from build123d import *

# Parameters (mm, degrees)
F0_W     = 195.58
F0_H     = 91.44
F1_DEPTH = 127
F2_W     = 50.8
F2_H     = 91.44
F3_DEPTH = 123.19


with BuildPart() as f1:
    # F0 (on Front) → F1 (new body)
    with BuildSketch(Plane.XZ):
        with Locations((97.79, 45.72)):
            Rectangle(F0_W, F0_H)
    extrude(amount=-F1_DEPTH)

    # F2 (on face) → F3 (cut)
    with BuildSketch(Plane.XZ):
        with Locations((25.4, 45.72)):
            Rectangle(F2_W, F2_H)
        with Locations((170.18, 45.72)):
            Rectangle(F2_W, F2_H)
    extrude(amount=-F3_DEPTH, mode=Mode.SUBTRACT)


solid = f1.part
Check sheet for the modelled part. Datum: model origin and axes. Units: mm. A direction names the side the tool comes from. Round coordinates to 2 decimals unless told otherwise and drop trailing zeros. Order: outer loops, then holes, each group sorted by start corner. A loop starts at its lowest first (then second) coordinate and runs counter-clockwise, first axis right, second up.
Q1. Depth check by flat-ended pin: P1, Ø15, axis at x = 31, z = 28, coming from the -Y side; P2, Ø4, axis at y = 40, z = 35.5, coming from the -X side. Enter the tip coordinate at first touch or a pass-through.
Filled sheet:
P1: stops at y = 123.19
P2: stops at x = 50.8
Q2. Scan lines: L1, parallel to Y at x = 152, z = 73.5; L2, parallel to X at y = 94, z = 65.5. Record each from-to range of solid material in increasing order.
Filled sheet:
L1: y = 123.19 to 127
L2: x = 50.8 to 144.78
Q3. Cross-section at C-C, the plane x = 169.5. Enter the section's corners in (y, z), plus the area to 3 significant figures.
Filled sheet:
outline: (123.19, 0) - (127, 0) - (127, 91.44) - (123.19, 91.44) - close
area: 348 mm2
Q4. Cross-section at A-A, the plane z = 29.5. Enter the section's corners in (x, y), plus the area to 3 significant figures.
Filled sheet:
outline: (0, 123.19) - (50.8, 123.19) - (50.8, 0) - (144.78, 0) - (144.78, 123.19) - (195.58, 123.19) - (195.58, 127) - (0, 127) - close
area: 12,300 mm2
Q5. Cross-section at B-B, the plane y = 104. Enter the section's corners in (x, z).
Filled sheet:
outline: (50.8, 0) - (144.78, 0) - (144.78, 91.44) - (50.8, 91.44) - close
Q6. Set-up check for faces 1 (the face through (50.8, 61, 45)), 2 (the face through (144.78, 61, 45)), 3 (the face through (96, 127, 46)): record each of +Z, -Z, +X, -X, +Y, -Y from which the full face is reachable in a straight line by a thin tool's end or side.
Filled sheet:
face 1: +Z, -Z, -X, -Y
face 2: +Z, -Z, +X, -Y
face 3: +Z, -Z, +X, -X, +Y
